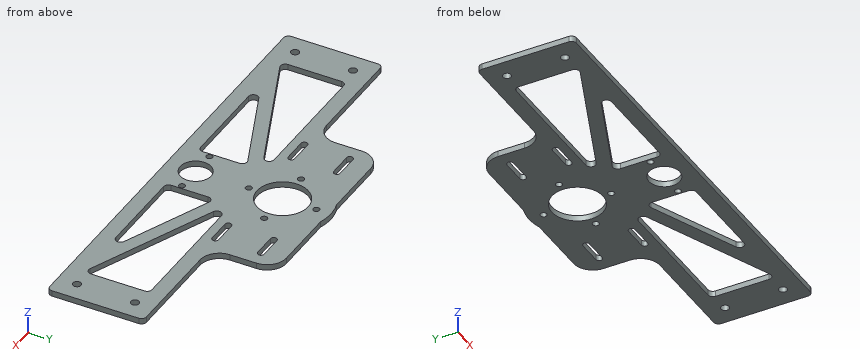
```python
from build123d import *

# Parameters (mm, degrees)
SKETCH_1_R          = 13.25
SKETCH_1_R_2        = 1.65
SKETCH_1_R_3        = 2.1
SKETCH_1_R_4        = 8
EXTRUDE_1_DEPTH     = 3
FILLET_1_R          = 10
CUT_EXTRUDE_1_DEPTH = 3
FILLET_3_R          = 2.5
SKETCH_3_R          = 1.65
CUT_EXTRUDE_2_DEPTH = 129.418261941
CUT_EXTRUDE_3_DEPTH = 129.418261941


with BuildPart() as part:
    # 草图1 → 凸台-拉伸1 (new body)
    with BuildSketch(Plane.XY):
        with BuildLine():
            Line((113.5, -10), (113.5, -60))
            Line((113.5, -60), (-113.5, -60))
            Line((-113.5, -60), (-113.5, -10))
            Line((-113.5, -10), (-50, -10))
            Line((-50, -10), (-50, 23.815246989))
            Line((-50, 23.815246989), (-7.604867576, 23.815246989))
            ThreePointArc((-7.604867576, 23.815246989), (0, 25), (7.604867576, 23.815246989))
            Line((7.604867576, 23.815246989), (50, 23.815246989))
            Line((50, 23.815246989), (50, -10))
            Line((50, -10), (113.5, -10))
        make_face()
        Circle(SKETCH_1_R, mode=Mode.SUBTRACT)
        with Locations((0, 17.5)):
            Circle(SKETCH_1_R_2, mode=Mode.SUBTRACT)
        with Locations((-17.5, 0)):
            Circle(SKETCH_1_R_2, mode=Mode.SUBTRACT)
        with Locations((0, -17.5)):
            Circle(SKETCH_1_R_2, mode=Mode.SUBTRACT)
        with Locations((17.5, 0)):
            Circle(SKETCH_1_R_2, mode=Mode.SUBTRACT)
        with Locations((103.5, -20)):
            Circle(SKETCH_1_R_3, mode=Mode.SUBTRACT)
        with Locations((103.5, -50)):
            Circle(SKETCH_1_R_3, mode=Mode.SUBTRACT)
        with Locations((0, -45)):
            Circle(SKETCH_1_R_4, mode=Mode.SUBTRACT)
        with Locations(Location((-103.5, -50, 0), (0, 0, 180))):
            Circle(SKETCH_1_R_3, mode=Mode.SUBTRACT)
        with Locations(Location((-103.5, -20, 0), (0, 0, 180))):
            Circle(SKETCH_1_R_3, mode=Mode.SUBTRACT)
    extrude(amount=EXTRUDE_1_DEPTH)

    # 圆角1
    fillet_1_edges = [part.edges().sort_by_distance(p)[0] for p in [
        (50, 23.815246989, 1.5),
        (50, -10, 1.5),
        (-50, -10, 1.5),
        (-50, 23.815246989, 1.5),
    ]]
    fillet(fillet_1_edges, radius=FILLET_1_R)

    # 草图2 → 切除-拉伸1 (cut)
    with BuildSketch(Plane.XY.offset(3)):
        Polygon((-93.5, -18), (-93.5, -52), (-12.5, -18), align=None)
        Polygon((12.5, -18), (93.5, -18), (93.5, -52), align=None)
        Polygon((-75.413964744, -52), (-15, -26.641051836), (-15, -52), align=None)
        Polygon((15, -52), (75.413964744, -52), (15, -26.641051836), align=None)
    extrude(amount=-CUT_EXTRUDE_1_DEPTH, mode=Mode.SUBTRACT)

    # 圆角3
    fillet_3_edges = [part.edges().sort_by_distance(p)[0] for p in [
        (-15, -52, 1.5),
        (-75.413964744, -52, 1.5),
        (-15, -26.641051836, 1.5),
        (15, -52, 1.5),
        (15, -26.641051836, 1.5),
        (75.413964744, -52, 1.5),
        (93.5, -52, 1.5),
        (12.5, -18, 1.5),
        (93.5, -18, 1.5),
        (-93.5, -18, 1.5),
        (-12.5, -18, 1.5),
        (-93.5, -52, 1.5),
        (113.5, -10, 1.5),
        (113.5, -60, 1.5),
        (-113.5, -60, 1.5),
        (-113.5, -10, 1.5),
    ]]
    fillet(fillet_3_edges, radius=FILLET_3_R)

    # 草图3 → 切除-拉伸2 (cut, through all)
    with BuildSketch(Plane.XY.offset(3)):
        with Locations((-13, -45)):
            Circle(SKETCH_3_R)
        with Locations((13, -45)):
            Circle(SKETCH_3_R)
    extrude(amount=-CUT_EXTRUDE_2_DEPTH, mode=Mode.SUBTRACT)

    # 草图4 → 切除-拉伸3 (cut, through all)
    with BuildSketch(Plane.XY.offset(3)):
        with BuildLine():
            Line((-42.2, 13.45), (-30, 13.45))
            ThreePointArc((-30, 13.45), (-28.35, 11.8), (-30, 10.15))
            Line((-30, 10.15), (-42.2, 10.15))
            ThreePointArc((-42.2, 10.15), (-43.85, 11.8), (-42.2, 13.45))
        make_face()
        with BuildLine():
            Line((-42.2, -13.45), (-30, -13.45))
            ThreePointArc((-30, -13.45), (-28.35, -11.8), (-30, -10.15))
            Line((-30, -10.15), (-42.2, -10.15))
            ThreePointArc((-42.2, -10.15), (-43.85, -11.8), (-42.2, -13.45))
        make_face()
        with BuildLine():
            Line((42.2, 13.45), (30, 13.45))
            ThreePointArc((30, 13.45), (28.35, 11.8), (30, 10.15))
            Line((30, 10.15), (42.2, 10.15))
            ThreePointArc((42.2, 10.15), (43.85, 11.8), (42.2, 13.45))
        make_face()
        with BuildLine():
            Line((42.2, -13.45), (30, -13.45))
            ThreePointArc((30, -13.45), (28.35, -11.8), (30, -10.15))
            Line((30, -10.15), (42.2, -10.15))
            ThreePointArc((42.2, -10.15), (43.85, -11.8), (42.2, -13.45))
        make_face()
    extrude(amount=-CUT_EXTRUDE_3_DEPTH, mode=Mode.SUBTRACT)


solid = part.part
```
Can you work these out from the model? Positions are in its coordinate system, mm. Round coordinates to 2 decimals unless told otherwise and drop trailing zeros. Loops run counter-clockwise (first coordinate to the right, second up) from the corner with the lowest first, then second, coordinate; pieces in that order, holes last. Notation, with made-up numbers: M 51,9 L 98,9 A37 ccw 98,48 Z; hole C 68.25,68 d5. An arc over 180 degrees is marked long. Answer in a Markdown table with one row per item.
1. If we section it at D-D, the plane z = 0.9: Give the number of separate pieces and of enclosed holes in the cut face, plus the area to 3 significant figures.
Established:
| item | result |
|---|---|
| separate pieces | 1 |
| enclosed holes | 20 |
| area | 9,510 mm² |
2. If we section it at C-C, the plane x = 34.5: Please give me the cut outline in (y, z).
Established:
| item | result |
|---|---|
| outline | M -60,0 L -52,0 L -52,3 L -60,3 Z; M -34.83,0 L -27.23,0 L -27.23,3 L -34.83,3 Z; M -18,0 L -13.45,0 L -13.45,3 L -18,3 Z; M -10.15,0 L 10.15,0 L 10.15,3 L -10.15,3 Z; M 13.45,0 L 23.82,0 L 23.82,3 L 13.45,3 Z |
3. I'm going to push flat-ended pins straight in: pin 1 Ø2 at (x, y) = (13, -45) entering from +Z; pin 2 Ø1.5 at (x, z) = (-50, 2) entering from +Y; pin 3 Ø0.9 at (x, z) = (38.5, 2) entering from +Y. Where does each tip first touch, or does it pass through?
Established:
| item | result |
|---|---|
| pin 1 | through |
| pin 2 | y = 17.61 |
| pin 3 | y = 23.82 |
4. If we section it at A-A, the plane x = -103.5: Please give me the cut outline in (y, z), plus the area to 3 significant figures.
Established:
| item | result |
|---|---|
| outline | M -60,0 L -52.1,0 L -52.1,3 L -60,3 Z; M -47.9,0 L -22.1,0 L -22.1,3 L -47.9,3 Z; M -17.9,0 L -10,0 L -10,3 L -17.9,3 Z |
| area | 125 mm² |
5. Please list where these lines run through material, in increasing order: line 1 (Y direction, x = -103.5, z = 0.7); line 2 (Y direction, x = 0, z = 2.15); line 3 (Y direction, x = -17.5, z = 1.8). Write a range as from..to.
Established:
| item | result |
|---|---|
| line 1 | -60..-52.1, -47.9..-22.1, -17.9..-10 |
| line 2 | -60..-53, -37..-19.15, -15.85..-13.25, 13.25..15.85, 19.15..25 |
| line 3 | -60..-52, -27.9..-1.65, 1.65..23.82 |
6. If we section it at B-B, the plane y = 4: Please give me the cut outline in (x, z).
Established:
| item | result |
|---|---|
| outline | M -50,0 L -12.63,0 L -12.63,3 L -50,3 Z; M 12.63,0 L 50,0 L 50,3 L 12.63,3 Z |
